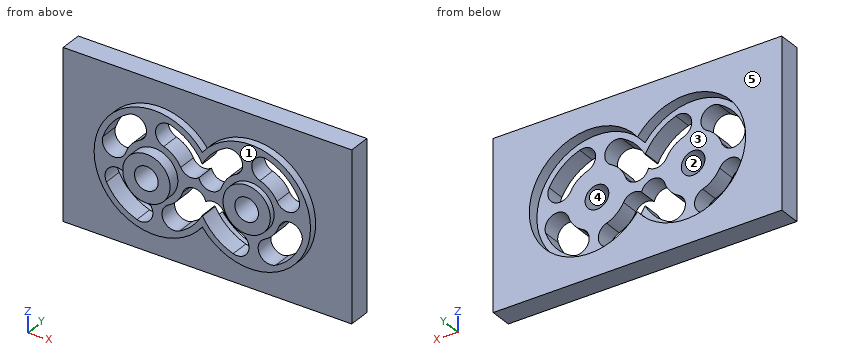
from build123d import *

# Parameters (mm, degrees)
F2_W          = 304.8
F2_H          = 177.8
F3_DEPTH      = 23.241
F0_R          = 25
F0_R_2        = 12.4968
F4_DEPTH      = 12.1666
F5_DEPTH      = 19.5326
F6_W          = 127
F6_H          = 25.4
F7_DEPTH      = 127
F7_DEPTH_BACK = 127
F9_DEPTH      = 31.243


with BuildPart() as f3:
    # F2 (on offset) → F3 (new body)
    with BuildSketch(Plane.XZ.offset(-31.242)):
        Rectangle(F2_W, F2_H)
        with BuildLine():
            ThreePointArc((0, -38.1), (-114.3, 0), (0, 38.1))
            ThreePointArc((0, 38.1), (70.8804631421, 60.2413894262), (114.3, 0))
            ThreePointArc((114.3, 0), (70.8804631421, -60.2413894262), (0, -38.1))
        make_face(mode=Mode.SUBTRACT)
    extrude(amount=F3_DEPTH)



with BuildPart() as f4:
    # F0 (on Front) → F4 (new body)
    with BuildSketch(Plane.XZ):
        with Locations((-50.8, 0)):
            Circle(F0_R)
        with Locations((-50.8, 0)):
            Circle(F0_R_2, mode=Mode.SUBTRACT)
    extrude(amount=F4_DEPTH)


with BuildPart() as f4b:
    # F0 (on Front) → F4, piece 2 (new body)
    with BuildSketch(Plane.XZ):
        with Locations((50.8, 0)):
            Circle(F0_R)
        with Locations((50.8, 0)):
            Circle(F0_R_2, mode=Mode.SUBTRACT)
    extrude(amount=F4_DEPTH)


with BuildPart() as f3_1:
    add(f3.part)

    add(f4.part)  # F5 merges F4

    add(f4b.part)  # F5 merges F4b
    # F0 (on Front) → F5 (join)
    with BuildSketch(Plane.XZ):
        with BuildLine():
            ThreePointArc((0, -38.1), (-12.7, 0), (0, 38.1))
            ThreePointArc((0, 38.1), (-114.3, 0), (0, -38.1))
        make_face()
        with Locations((-50.8, 0)):
            Circle(F0_R, mode=Mode.SUBTRACT)
        with Locations((-50.8, 0)):
            Circle(F0_R)
        with Locations((-50.8, 0)):
            Circle(F0_R_2, mode=Mode.SUBTRACT)
        with BuildLine():
            ThreePointArc((0, 38.1), (9.4413894262, 20.0804631421), (12.7, 0))
            ThreePointArc((12.7, 0), (9.4413894262, -20.0804631421), (0, -38.1))
            ThreePointArc((0, -38.1), (70.8804631421, -60.2413894262), (114.3, 0))
            ThreePointArc((114.3, 0), (70.8804631421, 60.2413894262), (0, 38.1))
        make_face()
        with Locations((50.8, 0)):
            Circle(F0_R, mode=Mode.SUBTRACT)
        with Locations((50.8, 0)):
            Circle(F0_R)
        with Locations((50.8, 0)):
            Circle(F0_R_2, mode=Mode.SUBTRACT)
        with BuildLine():
            ThreePointArc((0, -38.1), (9.4413894262, -20.0804631421), (12.7, 0))
            ThreePointArc((12.7, 0), (9.4413894262, 20.0804631421), (0, 38.1))
            ThreePointArc((0, 38.1), (-12.7, 0), (0, -38.1))
        make_face()
    extrude(amount=-F5_DEPTH)

    # F6 (on Top) → F7 (cut, two sides)
    with BuildSketch(Plane.XY) as f7_sk:
        with Locations((63.5, -18.5166)):
            Rectangle(F6_W, F6_H)
    extrude(amount=-F7_DEPTH, mode=Mode.SUBTRACT)
    extrude(f7_sk.sketch, amount=F7_DEPTH_BACK, mode=Mode.SUBTRACT)

    # F8 (on Front) → F9 (cut, through all)
    with BuildSketch(Plane.XZ):
        with BuildLine():
            ThreePointArc((-65.7271030045, 28.0222071917), (-60.4890613296, 45.2019312701), (-77.6687854081, 50.439972945))
            ThreePointArc((-77.6687854081, 50.439972945), (-94.411945371, 36.9340049406), (-104.9761603541, 18.1952232547))
            ThreePointArc((-104.9761603541, 18.1952232547), (-96.9803965542, 2.1126935639), (-80.8978668634, 10.1084573637))
            ThreePointArc((-80.8978668634, 10.1084573637), (-75.0288585395, 20.5188916337), (-65.7271030045, 28.0222071917))
        make_face()
        with BuildLine():
            ThreePointArc((-78.8222071917, -14.9271030045), (-96.0019312701, -9.6890613296), (-101.239972945, -26.8687854081))
            ThreePointArc((-101.239972945, -26.8687854081), (-87.7340049406, -43.611945371), (-68.9952232547, -54.1761603541))
            ThreePointArc((-68.9952232547, -54.1761603541), (-52.9126935639, -46.1803965542), (-60.9084573637, -30.0978668634))
            ThreePointArc((-60.9084573637, -30.0978668634), (-71.3188916337, -24.2288585395), (-78.8222071917, -14.9271030045))
        make_face()
        with BuildLine():
            ThreePointArc((-35.8728969955, -28.0222071917), (-41.1109386704, -45.2019312701), (-23.9312145919, -50.439972945))
            ThreePointArc((-23.9312145919, -50.439972945), (-10.107305041, -40.127634829), (0.010733032, -26.1608850911))
            ThreePointArc((0.010733032, -26.1608850911), (0.1798786546, -26.5175497593), (0.360027055, -26.8687854081))
            ThreePointArc((0.360027055, -26.8687854081), (13.8659950594, -43.611945371), (32.6047767453, -54.1761603541))
            ThreePointArc((32.6047767453, -54.1761603541), (48.6873064361, -46.1803965542), (40.6915426363, -30.0978668634))
            ThreePointArc((40.6915426363, -30.0978668634), (30.2811083663, -24.2288585395), (22.7777928083, -14.9271030045))
            ThreePointArc((22.7777928083, -14.9271030045), (14.1328150363, -8.4594398503), (3.6348708656, -10.9812399102))
            ThreePointArc((3.6348708656, -10.9812399102), (-8.2078269406, -1.4599992342), (-20.7021331366, -10.1084573637))
            ThreePointArc((-20.7021331366, -10.1084573637), (-26.5711414605, -20.5188916337), (-35.8728969955, -28.0222071917))
        make_face()
        with BuildLine():
            ThreePointArc((-0.010733032, 26.1608850911), (-0.1798786546, 26.5175497593), (-0.360027055, 26.8687854081))
            ThreePointArc((-0.360027055, 26.8687854081), (-13.8659950594, 43.611945371), (-32.6047767453, 54.1761603541))
            ThreePointArc((-32.6047767453, 54.1761603541), (-48.6873064361, 46.1803965542), (-40.6915426363, 30.0978668634))
            ThreePointArc((-40.6915426363, 30.0978668634), (-30.2811083663, 24.2288585395), (-22.7777928083, 14.9271030045))
            ThreePointArc((-22.7777928083, 14.9271030045), (-14.1328150363, 8.4594398503), (-3.6348708656, 10.9812399102))
            ThreePointArc((-3.6348708656, 10.9812399102), (8.2078269406, 1.4599992342), (20.7021331366, 10.1084573637))
            ThreePointArc((20.7021331366, 10.1084573637), (26.5711414605, 20.5188916337), (35.8728969955, 28.0222071917))
            ThreePointArc((35.8728969955, 28.0222071917), (41.1109386704, 45.2019312701), (23.9312145919, 50.439972945))
            ThreePointArc((23.9312145919, 50.439972945), (10.107305041, 40.127634829), (-0.010733032, 26.1608850911))
        make_face()
        with BuildLine():
            ThreePointArc((101.239972945, 26.8687854081), (87.7340049406, 43.611945371), (68.9952232547, 54.1761603541))
            ThreePointArc((68.9952232547, 54.1761603541), (52.9126935639, 46.1803965542), (60.9084573637, 30.0978668634))
            ThreePointArc((60.9084573637, 30.0978668634), (71.3188916337, 24.2288585395), (78.8222071917, 14.9271030045))
            ThreePointArc((78.8222071917, 14.9271030045), (96.0019312701, 9.6890613296), (101.239972945, 26.8687854081))
        make_face()
        with BuildLine():
            ThreePointArc((77.6687854081, -50.439972945), (94.411945371, -36.9340049406), (104.9761603541, -18.1952232547))
            ThreePointArc((104.9761603541, -18.1952232547), (96.9803965542, -2.1126935639), (80.8978668634, -10.1084573637))
            ThreePointArc((80.8978668634, -10.1084573637), (75.0288585395, -20.5188916337), (65.7271030045, -28.0222071917))
            ThreePointArc((65.7271030045, -28.0222071917), (60.4890613296, -45.2019312701), (77.6687854081, -50.439972945))
        make_face()
    extrude(amount=-F9_DEPTH, mode=Mode.SUBTRACT)


solid = f3_1.part
Source: CAD feature listing. Evaluate the final solid. Frame: model axes, mm. Face numbers are marked on the shaded views. A direction names the side the tool comes from. Round coordinates to 2 decimals unless told otherwise and drop trailing zeros. Loops run counter-clockwise (first coordinate to the right, second up) from the corner with the lowest first, then second, coordinate; pieces in that order, holes last. Notation, with made-up numbers: (-26.5, 14) - (14.5, 14) arc R33 ccw to (14.5, 42) - close; hole circle Ø8 at (75.25, 0.5). An arc over 180 degrees is marked (long way). Write item = value, one per line. Start each with the question number.
Item 1: Section query C-C on z = -69. Output: boundary loops of the cut face in (x, y).
Item 2: Section query B-B on x = -108.5. Output: boundary loops of the cut face in (y, z).
Item 3: Reachability of the marked faces 1, 2 and 3 from +Z, -Z, +X, -X, +Y, -Y: full face, straight path, thin tool, end or side. Return the list, or none.
Item 4: Material intervals for line 1 (X direction, y = 22, z = 0); line 2 (Z direction, x = 50.8, y = 0.75); line 3 (Z direction, x = -28, y = 16.5), sorted ascending.
Item 5: Section query A-A on x = 17.5. Output: boundary loops of the cut face in (y, z).
Item 6: Mould query, pull axis X, two halves, no side actions, for the marked faces 4 and 5. Classes: released by +X, released by -X, zero draft, split by the parting line, or undercut.
Item 7: First-contact query: pin 1 Ø8 at (x, z) = (-118, 23.5) entering from -Y; pin 2 Ø12 at (x, z) = (-69.5, 5) entering from +Y; pin 3 Ø5 at (y, z) = (1.5, -6) entering from +X. Flat tips, straight axial feed; report the tip coordinate or a pass-through.
Results list:
q1.outline = (-152.4, 8) - (152.4, 8) - (152.4, 31.24) - (-152.4, 31.24) - close
q2.outline = (0, -26.51) - (8, -26.51) - (8, -88.9) - (31.24, -88.9) - (31.24, -26.51) - (19.53, -26.51) - (19.53, 26.51) - (31.24, 26.51) - (31.24, 88.9) - (8, 88.9) - (8, 26.51) - (0, 26.51) - close
q3.face_1 = -Y
q3.face_2 = +Y, -Y
q3.face_3 = +Y
q4.line_1 = -152.4 to -114.3, 114.3 to 152.4
q4.line_2 = -63.5 to -12.5, 12.5 to 63.5
q4.line_3 = -88.9 to -51.79, -22.1 to 22.1, 52.4 to 88.9
q5.outline = (0, -54.07) - (8, -54.07) - (8, -88.9) - (31.24, -88.9) - (31.24, -54.07) - (19.53, -54.07) - (19.53, -46.45) - (0, -46.45) - close; (0, -9.67) - (19.53, -9.67) - (19.53, 5.03) - (0, 5.03) - close; (0, 46.45) - (19.53, 46.45) - (19.53, 54.07) - (31.24, 54.07) - (31.24, 88.9) - (8, 88.9) - (8, 54.07) - (0, 54.07) - close
q6.face_4 = undercut
q6.face_5 = zero draft
q7.pin_1 = 8
q7.pin_2 = 19.53
q7.pin_3 = 114.2
